```python
from build123d import *

# Parameters (mm, degrees)
SKETCH1_W                      = 58
SKETCH1_H                      = 35
BOSS_EXTRUDE1_DEPTH            = 2
M3X0_5_TAPPED_HOLE1_AT_2_COUNT = 2
M3X0_5_TAPPED_HOLE1_AT_2_PITCH = 20
M3X0_5_TAPPED_HOLE1_AT_3_COUNT = 2
M3X0_5_TAPPED_HOLE1_AT_3_PITCH = 39.8
M3X0_5_TAPPED_HOLE1_AT_4_COUNT = 2
M3X0_5_TAPPED_HOLE1_AT_4_PITCH = 44.102607633
M3X0_5_TAPPED_HOLE1_AT_5_COUNT = 2
M3X0_5_TAPPED_HOLE1_AT_5_PITCH = 14
CUT_EXTRUDE1_DEPTH             = 34.930075155
CHAMFER1_SIZE                  = 2


with BuildPart() as part:
    # Sketch1 → Boss-Extrude1 (new body)
    with BuildSketch(Plane(origin=(0, 0, 0), x_dir=(1, 0, 0), z_dir=(0, 1, 0))):
        Rectangle(SKETCH1_W, SKETCH1_H)
    extrude(amount=BOSS_EXTRUDE1_DEPTH)

    # Sketch3 → M3x0.5 Tapped Hole1 (revolve, cut)
    with BuildSketch(Plane(origin=(-23, 2, -12.5), x_dir=(0, 0, 1), z_dir=(1, 0, 0))):
        Polygon((0, 0), (0, 2), (1.75, 2), (1.75, -0.225), (1.525, 0), align=None)
    m3x0_5_tapped_hole1 = revolve(axis=Axis((-23, 8.35, -12.5), (0, -1, 0)), mode=Mode.SUBTRACT)

    # M3x0.5 Tapped Hole1 at 2: M3x0.5 Tapped Hole1 ×2
    with Locations(*[(i * M3X0_5_TAPPED_HOLE1_AT_2_PITCH, 0, 0) for i in range(1, M3X0_5_TAPPED_HOLE1_AT_2_COUNT)]):
        add(m3x0_5_tapped_hole1, mode=Mode.SUBTRACT)

    # M3x0.5 Tapped Hole1 at 3: M3x0.5 Tapped Hole1 ×2
    with Locations(*[(i * M3X0_5_TAPPED_HOLE1_AT_3_PITCH, 0, 0) for i in range(1, M3X0_5_TAPPED_HOLE1_AT_3_COUNT)]):
        add(m3x0_5_tapped_hole1, mode=Mode.SUBTRACT)

    # M3x0.5 Tapped Hole1 at 4: M3x0.5 Tapped Hole1 ×2
    with Locations(*[Vector(0.9024409697382602, 0, 0.4308135282670086) * (i * M3X0_5_TAPPED_HOLE1_AT_4_PITCH) for i in range(1, M3X0_5_TAPPED_HOLE1_AT_4_COUNT)]):
        add(m3x0_5_tapped_hole1, mode=Mode.SUBTRACT)

    # M3x0.5 Tapped Hole1 at 5: M3x0.5 Tapped Hole1 ×2
    with Locations(*[(0, 0, i * M3X0_5_TAPPED_HOLE1_AT_5_PITCH) for i in range(1, M3X0_5_TAPPED_HOLE1_AT_5_COUNT)]):
        add(m3x0_5_tapped_hole1, mode=Mode.SUBTRACT)

    # Sketch4 → Cut-Extrude1 (cut, through all)
    with BuildSketch(Plane(origin=(0, 2, 0), x_dir=(1, 0, 0), z_dir=(0, 1, 0))):
        with BuildLine():
            ThreePointArc((-8.0625, -3.279581743), (-11.75, -6.5), (-8.0625, -9.720418257))
            ThreePointArc((-8.0625, -9.720418257), (3, -6.5), (-8.0625, -3.279581743))
        make_face()
    extrude(amount=-CUT_EXTRUDE1_DEPTH, mode=Mode.SUBTRACT)

    # Chamfer1
    chamfer1_edges = [part.edges().sort_by_distance(p)[0] for p in [
        (29, 1, 17.5),
        (-29, 1, 17.5),
        (-29, 1, -17.5),
        (29, 1, -17.5),
    ]]
    chamfer(chamfer1_edges, length=CHAMFER1_SIZE)


solid = part.part
```
For this review, take the finished solid that the model builds, in its own axes (mm). A direction names the side the tool comes from. Give positions to 0.01 mm unless a question says otherwise; leave off trailing zeros. Write each loop counter-clockwise with the first axis right and the second up, starting at its lowest first coordinate (ties: lowest second). Pieces come first, ordered by that corner, then holes. Notation, with made-up numbers: M 0.5,7 L 23.5,7 A19 cw 23.5,38 Z; hole C -0.5,-33 d10. An arc over 180 degrees is marked long. Answer as a JSON object with one key per item and string values. Group by question number.
Item 1: Draft analysis for pull direction Z (two halves, no side actions). For faces 1 (the cylindrical face through (2.996, 1.014, 6.716)), 2 (the flat face through (0, 1, 17.5)), 3 (the flat face through (-29, 1, 0)), state which applies: +Z half, -Z half, draft (parallel to the pull), parting line (faces both ways), or undercut.
Item 2: Tool access review of faces 4 (the cylindrical face through (-11.75, 1.01, 6.42)), 5 (the flat face through (28, 1, -16.5)): name each direction out of +Z, -Z, +X, -X, +Y, -Y from which nothing blocks a thin tool from reaching the whole face with its end or side.
Item 3: Consider section A-A on x = -23. Write out the cut boundary in (y, z), plus the area to 3 significant figures.
Item 4: For probe 1 along X at (y, z) = (0.6, -12.5); probe 2 along Z at (x, y) = (-3, 1.7); probe 3 along Z at (x, y) = (-4, 1.3), list the stretches that pass through material, from the lowest coordinate up. Write a range as [from, to].
Item 5: Consider section B-B on z = 6.5. Write out the cut boundary in (x, y).
Item 6: Consider section D-D on y = 0.55. Write out the cut boundary in (x, z), plus the area to 3 significant figures.
Item 7: Consider section C-C on z = -12.5. Write out the cut boundary in (x, y).
Check result:
{
 "1": {"face 1": "undercut", "face 2": "+Z half", "face 3": "draft"},
 "2": {"face 4": "+Y, -Y", "face 5": "-Z, +X, +Y, -Y"},
 "3": {"outline": "M 0,-17.5 L 2,-17.5 L 2,-14.25 L 0,-14.25 Z; M 0,-10.75 L 2,-10.75 L 2,-0.25 L 0,-0.25 Z; M 0,3.25 L 2,3.25 L 2,17.5 L 0,17.5 Z", "area": "56.0 mm^2"},
 "4": {"probe 1": "x = [-29, -24.75], [-21.25, -4.75], [-1.25, 15.05], [18.55, 29]", "probe 2": "z = [-17.5, -14.25], [-10.75, 0.5], [12.5, 17.5]", "probe 3": "z = [-17.5, -13.94], [-11.06, 0.58], [12.42, 17.5]"},
 "5": {"outline": "M -29,0 L -11.75,0 L -11.75,2 L -29,2 Z; M 3,0 L 15.05,0 L 15.05,2 L 3,2 Z; M 18.55,0 L 29,0 L 29,2 L 18.55,2 Z"},
 "6": {"outline": "M -29,-15.5 L -27,-17.5 L 27,-17.5 L 29,-15.5 L 29,15.5 L 27,17.5 L -27,17.5 L -29,15.5 Z; hole C -23,-12.5 d3.5; hole C -23,1.5 d3.5; hole M -8.06,3.28 A6 ccw long -8.06,9.72 A3.25 ccw long Z; hole C -3,-12.5 d3.5; hole C 16.8,-12.5 d3.5; hole C 16.8,6.5 d3.5", "area": "1,850 mm^2"},
 "7": {"outline": "M -29,0 L -24.75,0 L -24.75,2 L -29,2 Z; M -21.25,0 L -4.75,0 L -4.75,2 L -21.25,2 Z; M -1.25,0 L 15.05,0 L 15.05,2 L -1.25,2 Z; M 18.55,0 L 29,0 L 29,2 L 18.55,2 Z"}
}
